Part print with two shaded views. Sizes in mm from the minimum x, y, z corner. Round coordinates to 2 decimals unless told otherwise and drop trailing zeros. Order: outer loops, then holes, each group sorted by start corner. A loop starts at its lowest first (then second) coordinate and runs counter-clockwise, first axis right, second up. Notation, with made-up numbers: (40, -36) -> (59, -36) arc R12 cw to (59, -22) -> close; hole circle Ø5 at (77.5, 43). An arc over 180 degrees is marked (long way). Answer as a JSON object with one key per item and string values.
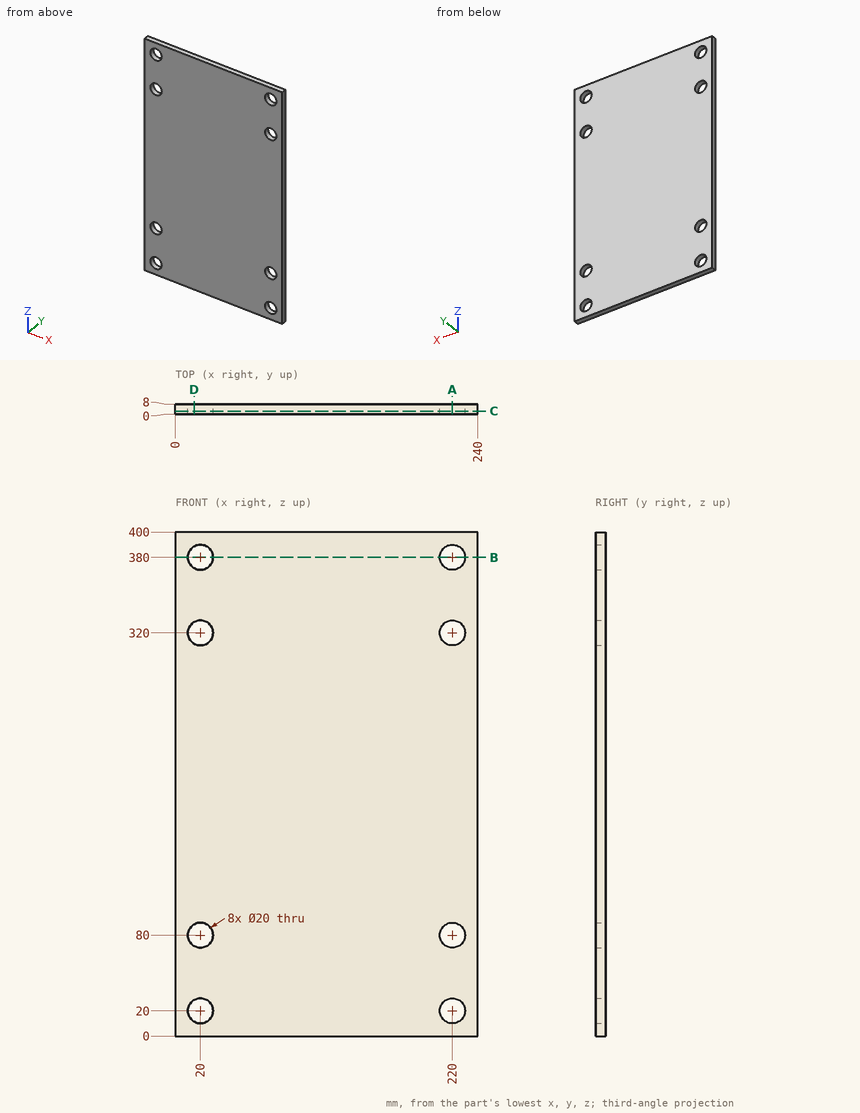
1) Cut at B-B, the plane z = 380. Give the cut face in (x, y).
Checked values:
{"outline": "(0, 0) -> (10, 0) -> (10, 8) -> (0, 8) -> close; (30, 0) -> (210, 0) -> (210, 8) -> (30, 8) -> close; (230, 0) -> (240, 0) -> (240, 8) -> (230, 8) -> close"}
2) Cut at A-A, the plane x = 220. Give the cut face in (y, z), plus the area to 3 significant figures.
Checked values:
{"outline": "(0, 0) -> (8, 0) -> (8, 10) -> (0, 10) -> close; (0, 30) -> (8, 30) -> (8, 70) -> (0, 70) -> close; (0, 90) -> (8, 90) -> (8, 310) -> (0, 310) -> close; (0, 330) -> (8, 330) -> (8, 370) -> (0, 370) -> close; (0, 390) -> (8, 390) -> (8, 400) -> (0, 400) -> close", "area": "2,560 mm²"}
3) Flat gauge pin, fed straight in: pin 1 Ø12 at (x, z) = (220, 20) entering from +Y. Where does the tip first touch, or does it go through?
Checked values:
{"pin 1": "passes through"}
4) Probe L1, parallel to X at y = 4.5, z = 319.5; L2, parallel to Z at x = 220, y = 2.25; L3, parallel to X at y = 4.75, z = 21. List the from-to ranges inside material, lowest first. Write a range as from..to.
Checked values:
{"L1": "x = 0..10.01, 29.99..210.01, 229.99..240", "L2": "z = 0..10, 30..70, 90..310, 330..370, 390..400", "L3": "x = 0..10.05, 29.95..210.05, 229.95..240"}
5) Cut at D-D, the plane x = 15. Give the cut face in (y, z), plus the area to 3 significant figures.
Checked values:
{"outline": "(0, 0) -> (8, 0) -> (8, 11.34) -> (0, 11.34) -> close; (0, 28.66) -> (8, 28.66) -> (8, 71.34) -> (0, 71.34) -> close; (0, 88.66) -> (8, 88.66) -> (8, 311.34) -> (0, 311.34) -> close; (0, 328.66) -> (8, 328.66) -> (8, 371.34) -> (0, 371.34) -> close; (0, 388.66) -> (8, 388.66) -> (8, 400) -> (0, 400) -> close", "area": "2,650 mm²"}
6) Cut at C-C, the plane y = 2.25. Count the separate pieces of the cut face and the enclosed holes in it, plus the area to 3 significant figures.
Checked values:
{"separate pieces": "1", "enclosed holes": "8", "area": "93,500 mm²"}
